For this review, use the dimensioned drawing (mm, ordinates from the lowest corner) and the shaded views. A direction names the side the tool comes from. Round coordinates to 2 decimals unless told otherwise and drop trailing zeros. Order: outer loops, then holes, each group sorted by start corner. A loop starts at its lowest first (then second) coordinate and runs counter-clockwise, first axis right, second up. Notation, with made-up numbers: M -30,-6 L 2,-6 A28 cw 2,22 Z; hole C 85.25,80.25 d1. An arc over 180 degrees is marked long. Answer as CSV lines item,"result". Start each with the question number.
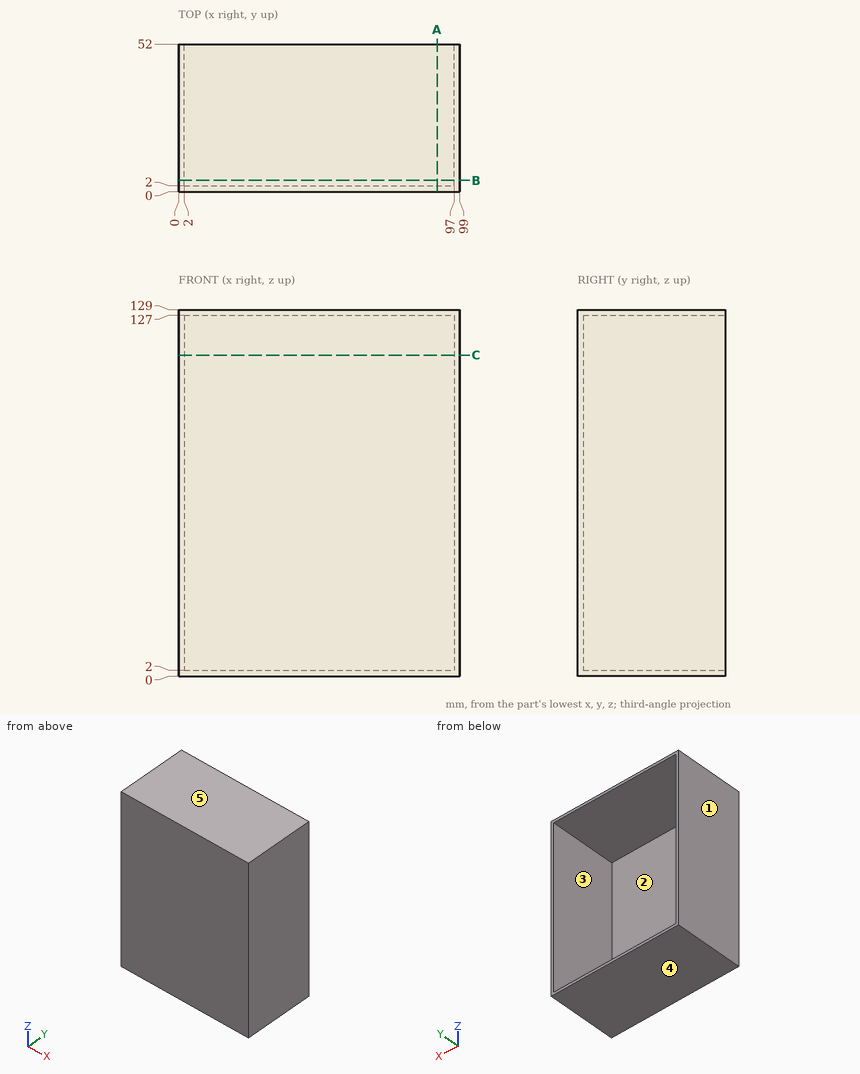
Item 1: Wall thickness on probe 1 along Z at (x, y) = (95, 20); probe 2 along X at (y, z) = (9, 99); probe 3 along Y at (x, z) = (39, 81): over which ranges is each line inside the solid? List them lowest first. Write a range as [from, to].
Item 2: Consider section C-C (z = 113). State the section outline as (x, y) points, and give its area (3 significant figures).
Item 3: Consider section A-A (x = 91). State the section outline as (y, z) points.
Item 4: Tool access review of the marked faces 1 and 2: name each direction out of +Z, -Z, +X, -X, +Y, -Y from which nothing blocks a thin tool from reaching the whole face with its end or side.
Item 5: Consider section B-B (y = 4). State the section outline as (x, z) points, and give its area (3 significant figures).
Item 6: For pin 1 (3 mm diameter, centred on x = 84, z = 68.5, fed in from +Y), flat-tipped, find the tip position at first contact; note if it passes through.
Item 7: The part is to be moulded in two halves that separate along Z. For the marked faces 3, 4 and 5, say which applies: +Z half, -Z half, draft (parallel to the pull), parting line (faces both ways), or undercut.
Reported:
1,probe 1,"z = [0, 2], [127, 129]"
1,probe 2,"x = [0, 2], [97, 99]"
1,probe 3,"y = [0, 2]"
2,outline,"M 0,0 L 99,0 L 99,52 L 97,52 L 97,2 L 2,2 L 2,52 L 0,52 Z"
2,area,"398 mm²"
3,outline,"M 0,0 L 52,0 L 52,2 L 2,2 L 2,127 L 52,127 L 52,129 L 0,129 Z"
4,face 1,"+Z, -Z, -X, +Y, -Y"
4,face 2,"+Y"
5,outline,"M 0,0 L 99,0 L 99,129 L 0,129 Z; hole M 2,2 L 97,2 L 97,127 L 2,127 Z"
5,area,"896 mm²"
6,pin 1,"stops at y = 2"
7,face 3,"undercut"
7,face 4,"-Z half"
7,face 5,"+Z half"
